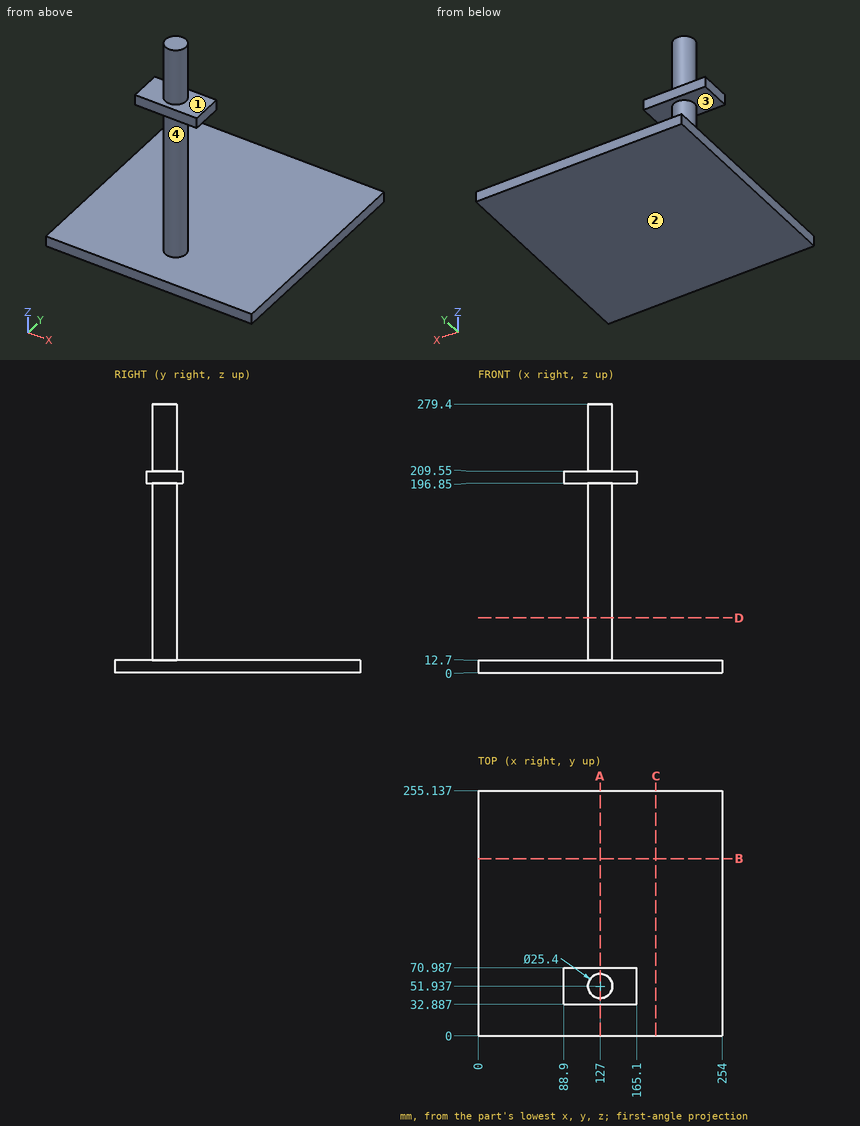
Here's the drawing with two shaded views (mm, measured from the low corner). I have some questions. Round coordinates to 2 decimals unless told otherwise and drop trailing zeros. Loops run counter-clockwise (first coordinate to the right, second up) from the corner with the lowest first, then second, coordinate; pieces in that order, holes last.
Item 1: Please list where these lines run through material, in increasing order: L1, parallel to Z at x = 236, y = 14; L2, parallel to Y at x = 126, z = 160; L3, parallel to Y at x = 141, z = 199.
Item 2: Suppose I cut it at C-C, the plane x = 185. Write out the boundary of the cut face in (y, z).
Item 3: Suppose I cut it at A-A, the plane x = 127. Write out the boundary of the cut face in (y, z).
Item 4: Suppose I cut it at B-B, the plane y = 184.5. Write out the boundary of the cut face in (x, z).
Item 5: Will these pins go through, and if not, where does the flat tip stop? pin 1 Ø4 at (y, z) = (42.5, 201.5) entering from +X; pin 2 Ø1 at (x, y) = (149.5, 54) entering from +Z; pin 3 Ø10 at (y, z) = (60.5, 206) entering from -X.
Item 6: Suppose I cut it at D-D, the plane z = 57. Write out the boundary of the cut face in (x, y), then the cut area to 3 significant figures.
Item 7: If we mould it in two halves opening along Z, with no side actions, what happens to the marked faces 1, 2, 3 and 4? For each: +Z half, -Z half, draft (parallel to the pull), parting line (faces both ways), or undercut.
Reported:
1. L1: z = 0 to 12.7
1. L2: y = 39.28 to 64.6
1. L3: y = 32.89 to 70.99
2. outline: (0, 0) - (255.14, 0) - (255.14, 12.7) - (0, 12.7) - close
3. outline: (0, 0) - (255.14, 0) - (255.14, 12.7) - (64.64, 12.7) - (64.64, 196.85) - (70.99, 196.85) - (70.99, 209.55) - (64.64, 209.55) - (64.64, 279.4) - (39.24, 279.4) - (39.24, 209.55) - (32.89, 209.55) - (32.89, 196.85) - (39.24, 196.85) - (39.24, 12.7) - (0, 12.7) - close
4. outline: (0, 0) - (254, 0) - (254, 12.7) - (0, 12.7) - close
5. pin 1: stops at x = 165.1
5. pin 2: stops at z = 209.55
5. pin 3: stops at x = 88.9
6. outline: circle Ø25.4 at (127, 51.94)
6. area: 507 mm2
7. face 1: +Z half
7. face 2: -Z half
7. face 3: undercut
7. face 4: undercut
